Input: part model. Units: mm. Frame: model coordinates. Round coordinates to 2 decimals unless told otherwise and drop trailing zeros. Order: outer loops, then holes, each group sorted by start corner. A loop starts at its lowest first (then second) coordinate and runs counter-clockwise, first axis right, second up. Notation, with made-up numbers: M 14,5 L 24,5 A27 ccw 24,33 Z; hole C 42,6 d2. An arc over 180 degrees is marked long. One line per question, with ' | ' between items.
Autodesk Inventor part; units mm, degrees
ref_plane "YZ Plane" through (0, 0, 0) normal (1, 0, 0) x (0, 1, 0)
ref_plane "XZ Plane" through (0, 0, 0) normal (0, 1, 0) x (-1, 0, 0)
ref_plane "XY Plane" through (0, 0, 0) normal (0, 0, 1) x (1, 0, 0)
sketch "Sketch1" plane through (0, 0, 0) normal (0, 0, 1) x (1, 0, 0)
  circle A0 centre (5.5, 0) radius 1.4795
  circle A1 centre (32.1927, 21.5482) radius 1.25
  circle A2 centre (5.5, 0) radius 3
  circle A3 centre (32.1927, 21.5482) radius 3
  point P0 (0, 0)
  dimension "d0" = 6
extrude "Extrusion1" add sketch "Sketch1" along normal blind 1
sketch "Sketch2" plane through (5.5, 0, 1) normal (0, 0, 1) x (1, 0, 0)
  circle A0 centre (0, 0) radius 3
  circle A1 centre (0, 0) radius 1.4795
  circle A2 centre (26.6927, 21.5482) radius 3
  circle A3 centre (26.6927, 21.5482) radius 1.25
  circle A4 centre (26.6927, 21.5482) radius 1.25
  arc A5 (0, 0) -> (26.6927, 21.5482) centre (-4.3622, 32.7104) ccw construction
  arc A6 (0.3966, -2.9737) -> (29.5159, 20.5335) centre (-4.3622, 32.7104) ccw
  arc A7 (-0.3966, 2.9737) -> (23.8695, 22.563) centre (-4.3622, 32.7104) ccw
  arc A8 (-0.3966, 2.9737) -> (0.3966, -2.9737) centre (0, 0) ccw
  arc A9 (29.5159, 20.5335) -> (23.8695, 22.563) centre (26.6927, 21.5482) ccw
  circle A10 centre (19.7, 21.8678) radius 2.5
  circle A11 centre (0, 0) radius 3
  point P0 (-5.5, 0)
  point P1 (23.8695, 22.563)
  point P2 (-0.3966, 2.9737)
  point P3 (0.3966, -2.9737)
  point P4 (29.5159, 20.5335)
  dimension "d3" = 30
extrude "Extrusion2" add sketch "Sketch2" along normal blind 3 contours A0 | A0 A7 A2 A6 | A2
sketch "Sketch3" plane through (5.5, 0, 1) normal (0, 0, -1) x (-1, 0, 0)
  arc A0 (-29.5159, 20.5335) -> (-23.8695, 22.563) centre (-26.6927, 21.5482) ccw construction
  arc A1 (-29.5159, 20.5335) -> (-0.3966, -2.9737) centre (4.3622, 32.7104) ccw construction
  arc A2 (0.3966, 2.9737) -> (-0.3966, -2.9737) centre (0, 0) ccw construction
  arc A3 (-23.8695, 22.563) -> (0.3966, 2.9737) centre (4.3622, 32.7104) ccw construction
  circle A4 centre (0, 0) radius 3 construction
  circle A5 centre (0, 0) radius 1.4795 construction
  arc A6 (-1, 0.149) -> (1, -0.1179) centre (4.3622, 32.7104) ccw construction
  arc A7 (-1.4875, -2.8111) -> (0.6943, -3.1022) centre (4.3622, 32.7104) ccw
  arc A8 (-0.5125, 3.1091) -> (1.3057, 2.8665) centre (4.3622, 32.7104) ccw
  arc A9 (-0.5125, 3.1091) -> (-1.4875, -2.8111) centre (-1, 0.149) ccw
  arc A10 (0.6943, -3.1022) -> (1.3057, 2.8665) centre (1, -0.1179) ccw
  point P0 (5.5, 0)
  dimension "d6" = 1
  dimension "d7" = 1
extrude "Extrusion3" add sketch "Sketch3" along normal blind 1 and the other way blind 4
sketch "Sketch4" plane through (5.5, 0, 4) normal (0, 0, 1) x (1, 0, 0)
  arc A0 (29.5159, 20.5335) -> (23.8695, 22.563) centre (26.6927, 21.5482) ccw
  circle A1 centre (26.6927, 21.5482) radius 1.25
  circle A2 centre (26.6927, 21.5482) radius 3
  circle A3 centre (26.6927, 21.5482) radius 3
  point P0 (-5.5, 0)
extrude "Extrusion4" add sketch "Sketch4" along normal blind 1
sketch "Sketch5" plane through (0, 0, 0) normal (0, 0, -1) x (-1, 0, 0)
  arc A0 (-6.9875, -2.8111) -> (-4.8057, -3.1022) centre (-1.1378, 32.7104) ccw
  arc A1 (-4.8057, -3.1022) -> (-4.1943, 2.8665) centre (-4.5, -0.1179) ccw
  arc A2 (-6.0125, 3.1091) -> (-4.1943, 2.8665) centre (-1.1378, 32.7104) ccw
  arc A3 (-6.0125, 3.1091) -> (-6.9875, -2.8111) centre (-6.5, 0.149) ccw
  arc A4 (-6.5, 0.149) -> (-4.5, -0.1179) centre (-1.1378, 32.7104) ccw construction
  arc A5 (-6.7031, -1.0844) -> (-4.6274, -1.3614) centre (-1.1378, 32.7104) ccw
  arc A6 (-6.2969, 1.3824) -> (-4.3726, 1.1256) centre (-1.1378, 32.7104) ccw
  arc A7 (-6.2969, 1.3824) -> (-6.7031, -1.0844) centre (-6.5, 0.149) ccw
  arc A8 (-4.6274, -1.3614) -> (-4.3726, 1.1256) centre (-4.5, -0.1179) ccw
  arc A9 (-6.9875, -2.8111) -> (-4.8057, -3.1022) centre (-1.1378, 32.7104) ccw
  point P0 (0, 0)
  dimension "d14" = 2.5
extrude "Extrusion5" cut sketch "Sketch5" against normal blind 5 contours A7 A6 A8 A5
equation "\"d7\" = d6"
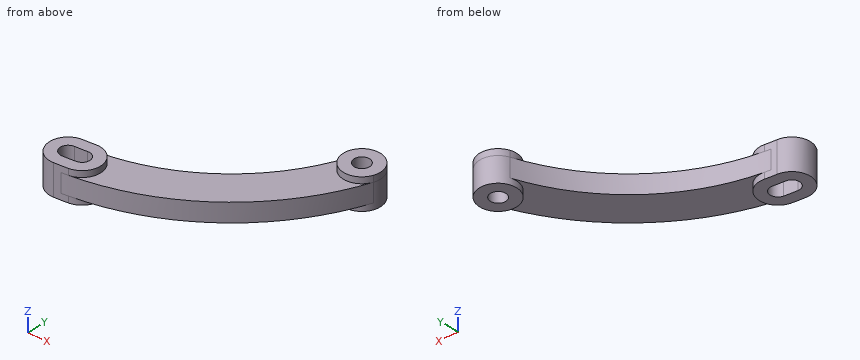
Item 1: Section query D-D, the plane x = 26. Return loops of the section in (y, z).
Report:
outline: M 6.67,1 L 15.92,1 L 15.92,4 L 6.67,4 Z
Item 2: Section query C-C, the plane z = 2.5. Return loops of the section in (x, y).
Report:
outline: M 4.19,2.87 A3 ccw 4.81,-3.1 A36 ccw 5.9,-2.97 A36 ccw 35.02,20.53 A3 ccw 29.37,22.56 A30 cw 5.1,2.97 A30.02 cw Z; hole M 4.37,1.13 A1.25 ccw 4.63,-1.36 A34.31 ccw 6.7,-1.08 A1.25 ccw 6.3,1.38 A31.81 cw Z; hole C 32.19,21.55 d2.5
Item 3: Section query A-A, the plane y = 0.25. Return loops of the section in (x, z).
Report:
outline: M 1.52,0 L 3.31,0 L 3.31,5 L 1.52,5 Z; M 7.75,0 L 9.5,0 L 9.5,1 L 16.7,1 L 16.7,4 L 9.5,4 L 9.5,5 L 7.75,5 Z
Item 4: Line query: line 1 along X through (y, z) = (0, 0.35); line 2 along Z through (x, y) = (9, 2.75); line 3 along X through (y, z) = (0, 2.45). Output: solid intervals per line, ascending. Write a range as from..to.
Report:
line 1: 1.5..3.26, 7.74..9.5 | line 2: 1..4 | line 3: 1.5..3.26, 7.74..16.17
Item 5: First-contact query: pin 1 (7.5 mm diameter, centred on x = 17, y = 6, fed in from +Z); pin 2 (2 mm diameter, centred on x = 6, z = 3, fed in from -Y); pin 3 (3 mm diameter, centred on x = 10.5, z = 2.5, fed in from -Y); pin 4 (3 mm diameter, centred on x = 32.19, y = 21.55, fed in from +Z). Flat tips, straight axial feed; report the tip coordinate or a pass-through.
Report:
pin 1: z = 4 | pin 2: y = -3.08 | pin 3: y = -2.42 | pin 4: z = 5
Item 6: Section query B-B, the plane z = 4.5. Return loops of the section in (x, y).
Report:
outline: M 4.19,2.87 A3 ccw 4.81,-3.1 A36 ccw 6.99,-2.81 A3 ccw 6.01,3.11 A30.02 cw Z; M 29.37,22.56 A3 ccw 35.02,20.53 A3 ccw Z; hole M 4.37,1.13 A1.25 ccw 4.63,-1.36 A34.31 ccw 6.7,-1.08 A1.25 ccw 6.3,1.38 A31.81 cw Z; hole C 32.19,21.55 d2.5
